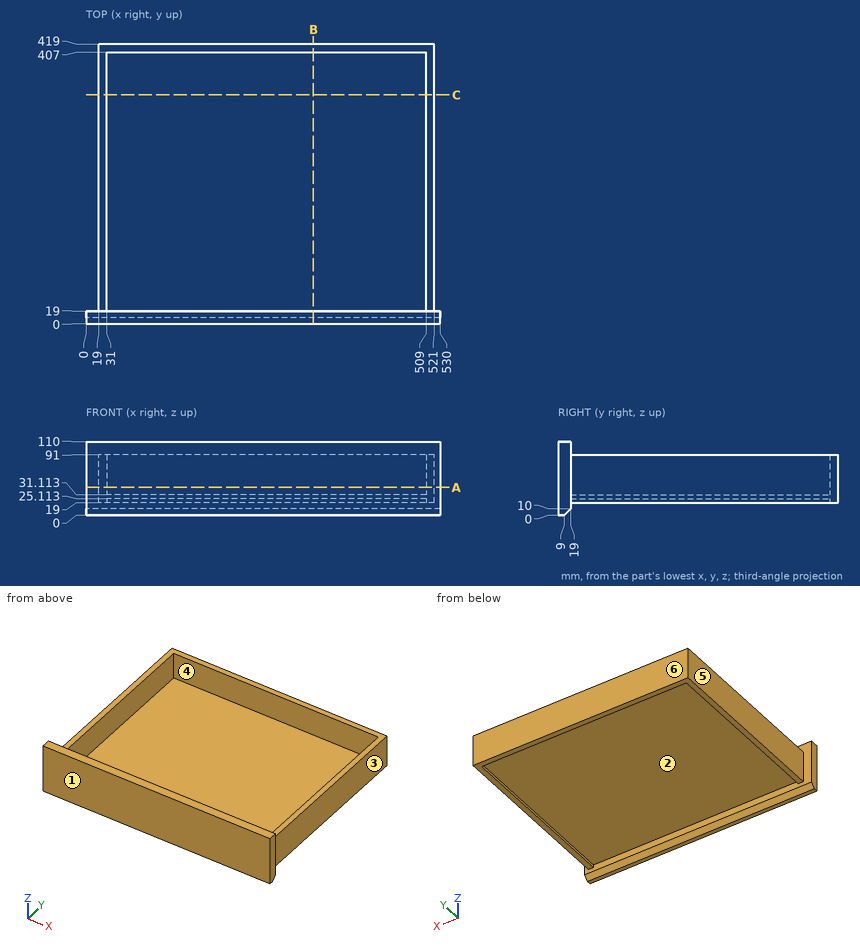
Design review of the part shown in the three views and the two pictorial views. Dimensions are in mm from the part's minimum x, y and z. A direction names the side the tool comes from. Round coordinates to 2 decimals unless told otherwise and drop trailing zeros. Loops run counter-clockwise (first coordinate to the right, second up) from the corner with the lowest first, then second, coordinate; pieces in that order, holes last. Notation, with made-up numbers: (78, 86) -> (132, 86) arc R21 cw to (132, 105) -> close; hole circle Ø1 at (32.25, 65). An arc over 180 degrees is marked (long way). Answer as CSV lines item,"result".
1) Draft analysis for pull direction X (two halves, no side actions). For the marked faces 1, 2 and 3, state which applies: pulls with the +X half, pulls with the -X half, needs draft (parallel to the pull), parting line crosses it, or undercut.
Geometry results:
face 1,"needs draft"
face 2,"undercut"
face 3,"pulls with the +X half"
2) To check wall thickness, follow line 1 along Y through (x, z) = (229, 50); line 2 along X through (y, z) = (136, 85.5); line 3 along Z through (x, y) = (40.5, 120.5). State the ranges of each line that lie inside material, in increasing order. Write a range as from..to.
Geometry results:
line 1,"y = 0..19, 407..419"
line 2,"x = 19..31, 509..521"
line 3,"z = 25.11..31.11"
3) Tool access review of the marked faces 4, 5 and 6: name each direction out of +Z, -Z, +X, -X, +Y, -Y from which nothing blocks a thin tool from reaching the whole face with its end or side.
Geometry results:
face 4,"+Z"
face 5,"+Z, -Z, -X, +Y"
face 6,"+Z, -Z, +X, -X, +Y"
4) Add section B-B on x = 340.5. Write out the cut boundary in (y, z).
Geometry results:
outline,"(0, 0) -> (9, 0) -> (19, 10) -> (19, 25.11) -> (407, 25.11) -> (407, 19) -> (419, 19) -> (419, 91) -> (407, 91) -> (407, 31.11) -> (19, 31.11) -> (19, 110) -> (0, 110) -> close"
5) For P1, Ø3, axis at y = 253.5, z = 36, coming from the +X side; P2, Ø3, axis at x = 218.5, z = 93.5, coming from the +Y side; P3, Ø3, axis at x = 100.5, y = 250.5, coming from the -Z side, all flat-tipped, find the tip position at first contact; note any pin that passes through.
Geometry results:
P1,"stops at x = 521"
P2,"stops at y = 19"
P3,"stops at z = 25.11"
6) Add section C-C on y = 343. Write out the cut boundary in (x, z), plus the area to 3 significant figures.
Geometry results:
outline,"(19, 19) -> (31, 19) -> (31, 25.11) -> (509, 25.11) -> (509, 19) -> (521, 19) -> (521, 91) -> (509, 91) -> (509, 31.11) -> (31, 31.11) -> (31, 91) -> (19, 91) -> close"
area,"4,600 mm²"
7) Add section A-A on z = 42. Write out the cut boundary in (x, y), plus the area to 3 significant figures.
Geometry results:
outline,"(0, 0) -> (530, 0) -> (530, 19) -> (521, 19) -> (521, 419) -> (19, 419) -> (19, 19) -> (0, 19) -> close; hole (31, 19) -> (509, 19) -> (509, 407) -> (31, 407) -> close"
area,"25,400 mm²"
